The listing builds one solid part. Answer for the finished solid, in the listing's coordinates (mm). A direction names the side the tool comes from. Round coordinates to 2 decimals unless told otherwise and drop trailing zeros. Loops run counter-clockwise (first coordinate to the right, second up) from the corner with the lowest first, then second, coordinate; pieces in that order, holes last. Notation, with made-up numbers: (-13, -39) -> (18, -39) arc R20 cw to (18, -21) -> close; hole circle Ø7 at (-0.5, 65.25). An arc over 180 degrees is marked (long way). Write each question's results on one line, items separated by ' | '. Start each with the question number.
(1) Determine the mould class of faces 6 (the face through (25.4, -67, 3)), 7 (the face through (35, -57.15, 3)), 8 (the face through (-54, -63.5, 3)) for opening direction Y: released by +Y, released by -Y, zero draft, split by the parting line, or undercut.
(2) The part is cut by section D-D (z = 4). Count the separate pieces of the cut face and the enclosed holes in it, plus the area to 3 significant figures.
(3) Straight lines are drawn through the part: probe 1 along X at (y, z) = (-52, 5.25); probe 2 along Y at (x, z) = (31, 1.75); probe 3 along Y at (x, z) = (-31.75, 2.5). For each, find the intervals that lie inside material, in ascending order.
(4) Flat-ended cylindrical pins translate along their axes: pin 1 (3 mm diameter, centred on y = -67.5, z = 4, fed in from +X); pin 2 (1.9 mm diameter, centred on y = -3.5, z = 2.5, fed in from +X); pin 3 (1.9 mm diameter, centred on x = 0.5, z = 4, fed in from -Y). Find the tip coordinate at first contact, or state that the pin passes through.
(5) The part is cut by section C-C (y = 44). Determine the outline of the cut face in (x, z).
(6) The part is cut by section B-B (x = -31.75). Determine the outline of the cut face in (y, z), plus the area to 3 significant figures.
(7) The part is cut by section A-A (y = -49). Determine the outline of the cut face in (x, z), plus the area to 3 significant figures.
(8) For faces 1 (the face through (67, 12.7, 3)), 2 (the face through (63.5, 51, 3)), 3 (the face through (57.15, -48, 3)), 4 (the face through (-60, 38.1, 3)), 5 (the face through (-25.4, -67, 3)), determine the directions among +Z, -Z, +X, -X, +Y, -Y from which every point of the face is accessible in a straight line to the end or side of a thin tool.
```python
from build123d import *

# Parameters (mm, degrees)
BOXSIDE_DEPTH      = 6.35
SKETCH2_R          = 3.96875
CUT_EXTRUDE1_DEPTH = 99.986703653
SKETCH3_W          = 44.45
SKETCH3_H          = 19.05
CUT_EXTRUDE2_DEPTH = 99.986703653
FILLET1_R          = 2.54


with BuildPart() as part:
    # Sketch1 → BOXSIDE (new body)
    with BuildSketch(Plane.XY):
        Polygon((-63.5, 38.1), (-63.5, 63.5), (63.5, 63.5), (63.5, 38.1), (69.85, 38.1), (69.85, 12.7), (63.5, 12.7), (63.5, -12.7), (69.85, -12.7), (69.85, -38.1), (63.5, -38.1), (63.5, -63.5), (44.45, -63.5), (44.45, -69.85), (25.4, -69.85), (25.4, -63.5), (-25.4, -63.5), (-25.4, -69.85), (-44.45, -69.85), (-44.45, -63.5), (-63.5, -63.5), (-63.5, -38.1), (-57.15, -38.1), (-57.15, -12.7), (-63.5, -12.7), (-63.5, 12.7), (-57.15, 12.7), (-57.15, 38.1), align=None)
    extrude(amount=BOXSIDE_DEPTH)

    # Sketch2 → Cut-Extrude1 (cut, through all)
    with BuildSketch(Plane.XY):
        with Locations(Location((-10.755250883, 25.77544668, 0), (0, 0, 180))):
            Circle(SKETCH2_R)
        with Locations((3.175, 0)):
            Circle(SKETCH2_R)
        with Locations((-31.75, 5.339056325)):
            Circle(SKETCH2_R)
    extrude(amount=CUT_EXTRUDE1_DEPTH, mode=Mode.SUBTRACT)

    # Sketch3 → Cut-Extrude2 (cut, through all)
    with BuildSketch(Plane(origin=(0, 0, 0), x_dir=(-1, 0, 0), z_dir=(0, 0, -1))):
        with Locations((-34.925, -47.625)):
            Rectangle(SKETCH3_W, SKETCH3_H)
    extrude(amount=-CUT_EXTRUDE2_DEPTH, mode=Mode.SUBTRACT)

    # Fillet1
    fillet1_edges = [part.edges().sort_by_distance(p)[0] for p in [
        (57.15, -57.15, 3.175),
        (57.15, -38.1, 3.175),
        (12.7, -38.1, 3.175),
        (12.7, -57.15, 3.175),
    ]]
    fillet(fillet1_edges, radius=FILLET1_R)


solid = part.part
```
Checked values:
1) face 6: zero draft | face 7: undercut | face 8: released by -Y
2) separate pieces: 1 | enclosed holes: 4 | area: 15,400 mm2
3) probe 1: x = -63.5 to 12.7, 57.15 to 63.5 | probe 2: y = -69.85 to -57.15, -38.1 to 63.5 | probe 3: y = -69.85 to 1.37, 9.31 to 63.5
4) pin 1: stops at x = 44.45 | pin 2: stops at x = 63.5 | pin 3: stops at y = -63.5
5) outline: (-63.5, 0) -> (63.5, 0) -> (63.5, 6.35) -> (-63.5, 6.35) -> close
6) outline: (-69.85, 0) -> (1.37, 0) -> (1.37, 6.35) -> (-69.85, 6.35) -> close; (9.31, 0) -> (63.5, 0) -> (63.5, 6.35) -> (9.31, 6.35) -> close | area: 796 mm2
7) outline: (-63.5, 0) -> (12.7, 0) -> (12.7, 6.35) -> (-63.5, 6.35) -> close; (57.15, 0) -> (63.5, 0) -> (63.5, 6.35) -> (57.15, 6.35) -> close | area: 524 mm2
8) face 1: +Z, -Z, +X | face 2: +Z, -Z, +X, +Y | face 3: +Z, -Z | face 4: +Z, -Z, -X | face 5: +Z, -Z, -Y
